Could you check a few things on this model? Use its own coordinates, in mm. Coordinates: 2 decimals unless noted, no trailing zeros. Order: outer loops, then holes, each group sorted by start corner. A loop starts at its lowest first (then second) coordinate and runs counter-clockwise, first axis right, second up. Notation, with made-up numbers: (30, 28.25) - (71, 28.25) arc R24 cw to (71, 63.25) - close; hole circle Ø4 at (40, 88). An arc over 180 degrees is marked (long way). One line per item, written item: value.
from build123d import *

# Parameters (mm, degrees)
SKETCH4_R           = 11.5
SKETCH4_R_2         = 1.5
BOSS_EXTRUDE1_DEPTH = 5
SKETCH5_R           = 1.5
CUT_EXTRUDE1_DEPTH  = 111.101739948


with BuildPart() as part:
    # Sketch4 → Boss-Extrude1 (new body)
    with BuildSketch(Plane.XY):
        with BuildLine():
            Line((-10.087403903, 107.088819702), (9.912596097, 107.088819702))
            ThreePointArc((9.912596097, 107.088819702), (20.519197815, 102.695421419), (24.912596097, 92.088819702))
            Line((24.912596097, 92.088819702), (24.912596097, 7.088819702))
            Line((24.912596097, 7.088819702), (-25.087403903, 7.088819702))
            Line((-25.087403903, 7.088819702), (-25.087403903, 92.088819702))
            ThreePointArc((-25.087403903, 92.088819702), (-20.694005621, 102.695421419), (-10.087403903, 107.088819702))
        make_face()
        with Locations((-0.087403903, 82.088819702)):
            Circle(SKETCH4_R, mode=Mode.SUBTRACT)
        with Locations((15.412596097, 66.588819702)):
            Circle(SKETCH4_R_2, mode=Mode.SUBTRACT)
        with Locations(Location((-15.587403903, 66.588819702, 0), (0, 0, 180))):
            Circle(SKETCH4_R_2, mode=Mode.SUBTRACT)
        with Locations(Location((15.412596097, 97.588819702, 0), (0, 0, 180))):
            Circle(SKETCH4_R_2, mode=Mode.SUBTRACT)
        with Locations((-15.587403903, 97.588819702)):
            Circle(SKETCH4_R_2, mode=Mode.SUBTRACT)
        with Locations((-8.087403903, 42.088819702)):
            Circle(SKETCH4_R_2, mode=Mode.SUBTRACT)
        with Locations(Location((7.912596097, 42.088819702, 0), (0, 0, 180))):
            Circle(SKETCH4_R_2, mode=Mode.SUBTRACT)
    extrude(amount=BOSS_EXTRUDE1_DEPTH)

    # Sketch5 → Cut-Extrude1 (cut, through all)
    with BuildSketch(Plane(origin=(0, 0, 0), x_dir=(-1, 0, 0), z_dir=(0, 0, -1))):
        with Locations((8.087403903, 26.088819702)):
            Circle(SKETCH5_R)
        with Locations((-7.912596097, 26.088819702)):
            Circle(SKETCH5_R)
    extrude(amount=-CUT_EXTRUDE1_DEPTH, mode=Mode.SUBTRACT)


solid = part.part
Item 1: I want a section at B-B on z = 2.2. Give the number of separate pieces and of enclosed holes in the cut face, then the cut area to 3 significant figures.
Conclusion:
separate pieces: 1
enclosed holes: 9
area: 4,430 mm²
Item 2: I want a section at A-A on x = 2.5. Please give me the cut outline in (y, z).
Conclusion:
outline: (7.09, 0) - (70.88, 0) - (70.88, 5) - (7.09, 5) - close; (93.29, 0) - (107.09, 0) - (107.09, 5) - (93.29, 5) - close
Item 3: If I drill on probe 1 along X at (y, z) = (82.5, 0.45); probe 2 along Y at (x, z) = (-7.5, 3.6); probe 3 along Y at (x, z) = (-16, 0.65), over which ranges is the centre line in solid material (lowest first)?
Conclusion:
probe 1: -25.09 to -11.58, 11.41 to 24.91
probe 2: 7.09 to 24.71, 27.47 to 40.71, 43.47 to 73.3, 90.88 to 107.09
probe 3: 7.09 to 65.15, 68.03 to 96.15, 99.03 to 105.87
Item 4: Thinking about a two-plate mould opening in X: for faces 1 (the face through (0, 58, 0)), 2 (the face through (-20.81, 102.58, 2.46)), 3 (the face through (9.103, 43.002, 2.465)), which applies, pulls with the +X half, pulls with the -X half, needs draft (parallel to the pull), parting line crosses it, or undercut?
Conclusion:
face 1: needs draft
face 2: pulls with the -X half
face 3: undercut
Item 5: I want a section at C-C on x = 19.5. Please give me the cut outline in (y, z), then the cut area to 3 significant figures.
Conclusion:
outline: (7.09, 0) - (103.62, 0) - (103.62, 5) - (7.09, 5) - close
area: 483 mm²
